Could you check a few things on this model? Use its own coordinates, in mm. Face numbers are marked on the shaded views. A direction names the side the tool comes from. Round coordinates to 2 decimals unless told otherwise and drop trailing zeros. Order: outer loops, then holes, each group sorted by start corner. A loop starts at its lowest first (then second) coordinate and runs counter-clockwise, first axis right, second up. Notation, with made-up numbers: (-14.75, 23) - (20.25, 23) arc R10 cw to (20.25, 35) - close; hole circle Ø9 at (2, 68). An arc over 180 degrees is marked (long way). Use one line per item in the form item = value.
from build123d import *

# Parameters (mm, degrees)
BOSS_EXTRUDE1_DEPTH = 12
SWEEP1_START        = 12
SWEEP1_DEPTH        = 4.545750983
SWEEP1_2_ANGLE      = 90
BOSS_EXTRUDE2_DEPTH = 170
SKETCH11_W          = 78
SKETCH11_H          = 58
CUT_EXTRUDE14_DEPTH = 10
SKETCH12_W          = 78
SKETCH12_H          = 58
CUT_EXTRUDE15_DEPTH = 10


with BuildPart() as part:
    # Sketch1 → Boss-Extrude1 (new body)
    with BuildSketch(Plane.XY):
        with BuildLine():
            Line((10, -28), (-10, -28))
            ThreePointArc((-10, -28), (-38, 0), (-10, 28))
            Line((-10, 28), (10, 28))
            ThreePointArc((10, 28), (38, 0), (10, -28))
        make_face()
        with BuildLine():
            Line((10, -25), (-10, -25))
            ThreePointArc((-10, -25), (-35, 0), (-10, 25))
            Line((-10, 25), (10, 25))
            ThreePointArc((10, 25), (35, 0), (10, -25))
        make_face(mode=Mode.SUBTRACT)
    extrude(amount=BOSS_EXTRUDE1_DEPTH)

    # Sweep1: read off the stored shape, not the designer's step
    # Sweep1 outline → Sweep1 (add)
    with BuildSketch(Plane.XY.offset(SWEEP1_START)):
        with BuildLine():
            ThreePointArc((-10, 28), (-38, 0), (-10, -28))
            Line((-10, -28), (10, -28))
            ThreePointArc((10, -28), (38, 0), (10, 28))
            Line((10, 28), (-10, 28))
        make_face()
        with BuildLine():
            Line((10, -25), (-10, -25))
            ThreePointArc((-10, -25), (-35, 0), (-10, 25))
            Line((-10, 25), (10, 25))
            ThreePointArc((10, 25), (35, 0), (10, -25))
        make_face(mode=Mode.SUBTRACT)
    extrude(amount=SWEEP1_DEPTH)

    # Sweep1 2 outline → Sweep1 2 (revolve)
    with BuildSketch(Plane(origin=(0, 28.510163598, 16.545750983), x_dir=(0, 0, 1), z_dir=(0, 1, 0))):
        with BuildLine():
            Line((0.510163598, 10), (0.510163598, -10))
            ThreePointArc((0.510163598, -10), (28.510163598, -38), (56.510163598, -10))
            Line((56.510163598, -10), (56.510163598, 10))
            ThreePointArc((56.510163598, 10), (28.510163598, 38), (0.510163598, 10))
        make_face()
        with BuildLine():
            Line((3.510163598, -10), (3.510163598, 10))
            ThreePointArc((3.510163598, 10), (28.510163598, 35), (53.510163598, 10))
            Line((53.510163598, 10), (53.510163598, -10))
            ThreePointArc((53.510163598, -10), (28.510163598, -35), (3.510163598, -10))
        make_face(mode=Mode.SUBTRACT)
    revolve(axis=Axis((0, 28.510163598, 16.545750983), (1, 0, 0)), revolution_arc=SWEEP1_2_ANGLE)

    # Sketch6 → Boss-Extrude2 (add)
    with BuildSketch(Plane(origin=(0, 28.510163598, 0), x_dir=(1, 0, 0), z_dir=(0, 1, 0))):
        with BuildLine():
            Line((10, -73.055914581), (-10, -73.055914581))
            ThreePointArc((-10, -73.055914581), (-38, -45.055914581), (-10, -17.055914581))
            Line((-10, -17.055914581), (10, -17.055914581))
            ThreePointArc((10, -17.055914581), (38, -45.055914581), (10, -73.055914581))
        make_face()
        with BuildLine():
            Line((10, -70.055914581), (-10, -70.055914581))
            ThreePointArc((-10, -70.055914581), (-35, -45.055914581), (-10, -20.055914581))
            Line((-10, -20.055914581), (10, -20.055914581))
            ThreePointArc((10, -20.055914581), (35, -45.055914581), (10, -70.055914581))
        make_face(mode=Mode.SUBTRACT)
    extrude(amount=BOSS_EXTRUDE2_DEPTH)

    # Sketch11 → Cut-Extrude14 (cut)
    with BuildSketch(Plane(origin=(0, 0, 0), x_dir=(-1, 0, 0), z_dir=(0, 0, -1))):
        Rectangle(SKETCH11_W, SKETCH11_H)
        with BuildLine():
            Line((10, -27), (-10, -27))
            ThreePointArc((-10, -27), (-37, 0), (-10, 27))
            Line((-10, 27), (10, 27))
            ThreePointArc((10, 27), (37, 0), (10, -27))
        make_face(mode=Mode.SUBTRACT)
    extrude(amount=-CUT_EXTRUDE14_DEPTH, mode=Mode.SUBTRACT)

    # Sketch12 → Cut-Extrude15 (cut)
    with BuildSketch(Plane(origin=(0, 198.510163598, 0), x_dir=(1, 0, 0), z_dir=(0, 1, 0))):
        with Locations((0, -45.055914581)):
            Rectangle(SKETCH12_W, SKETCH12_H)
        with BuildLine():
            Line((10, -72.055914581), (-10, -72.055914581))
            ThreePointArc((-10, -72.055914581), (-37, -45.055914581), (-10, -18.055914581))
            Line((-10, -18.055914581), (10, -18.055914581))
            ThreePointArc((10, -18.055914581), (37, -45.055914581), (10, -72.055914581))
        make_face(mode=Mode.SUBTRACT)
    extrude(amount=-CUT_EXTRUDE15_DEPTH, mode=Mode.SUBTRACT)


solid = part.part
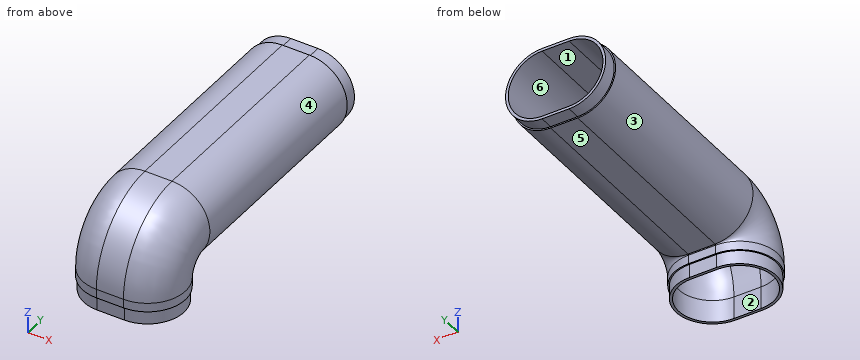
Item 1: Imagine slicing it at C-C on x = 16.5. Please give me the cut outline in (y, z).
Found:
outline = (-27.24, 10) - (-26.21, 10) - (-26.21, 0) - (-24.14, 0) - (-24.14, 16.55) arc R52.65 cw to (28.51, 69.2) - (198.51, 69.2) - (198.51, 71.26) - (188.51, 71.26) - (188.51, 72.29) - (28.51, 72.29) arc R55.75 ccw to (-27.24, 16.55) - close; (24.14, 0) - (26.21, 0) - (26.21, 10) - (27.24, 10) - (27.24, 16.55) arc R1.28 cw to (28.51, 17.82) - (188.51, 17.82) - (188.51, 18.85) - (198.51, 18.85) - (198.51, 20.92) - (28.51, 20.92) arc R4.37 ccw to (24.14, 16.55) - close
Item 2: Will these pins go through, and if not, where does the flat tip stop? P1, Ø4, axis at y = 7, z = 37.5, coming from the -X side; P2, Ø22, axis at x = -2, y = 74, coming from the -Z side; P3, Ø1.5, axis at y = 115.5, z = 27.5, coming from the -X side.
Found:
P1 = -38
P2 = 17.06
P3 = -32.4
Item 3: I need wall thicknesses on L1, parallel to Y at x = 2, z = 15.5; L2, parallel to Z at x = -1, y = 141; L3, parallel to Z at x = 23.5, y = 91.5. Which ranges of each line are inside material? Lowest first, please.
Found:
L1 = -28 to -25, 25 to 28
L2 = 17.06 to 20.06, 70.06 to 73.06
L3 = 20.53 to 24.01, 66.1 to 69.59
Item 4: Imagine slicing it at B-B on x = 6. Please give me the cut outline in (y, z).
Found:
outline = (-28, 10) - (-27, 10) - (-27, 0) - (-25, 0) - (-25, 16.55) arc R53.51 cw to (28.51, 70.06) - (198.51, 70.06) - (198.51, 72.06) - (188.51, 72.06) - (188.51, 73.06) - (28.51, 73.06) arc R56.51 ccw to (-28, 16.55) - close; (25, 0) - (27, 0) - (27, 10) - (28, 10) - (28, 16.55) arc R0.51 cw to (28.51, 17.06) - (188.51, 17.06) - (188.51, 18.06) - (198.51, 18.06) - (198.51, 20.06) - (28.51, 20.06) arc R3.51 ccw to (25, 16.55) - close
Item 5: For the marked faces 4, 5 and 6, which set-ups out of +Z, -Z, +X, -X, +Y, -Y let a thin tool reach every point of the face, with its end or its side?
Found:
face_4 = +X, +Y
face_5 = -Z, +X, -X, +Y
face_6 = +Y
Item 6: Imagine slicing it at A-A on y = 92. Please give me the cut outline in (x, z).
Found:
outline = (-10, 17.06) - (10, 17.06) arc R28 ccw to (10, 73.06) - (-10, 73.06) arc R28 ccw to start; hole (-10, 20.06) - (10, 20.06) arc R25 ccw to (10, 70.06) - (-10, 70.06) arc R25 ccw to start
Item 7: If we mould it in two halves opening along Z, with no side actions, what happens to the marked faces 1, 2 and 3? For each: released by +Z, released by -Z, zero draft, split by the parting line, or undercut.
Found:
face_1 = undercut
face_2 = zero draft
face_3 = split by the parting line
